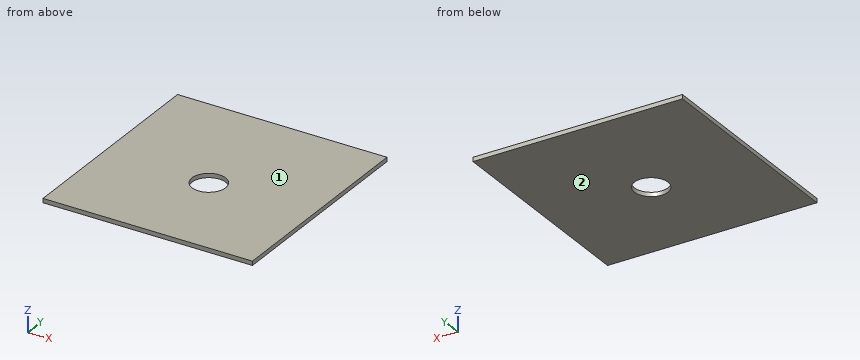
```python
from build123d import *

# Parameters (mm, degrees)
SKETCH1_W           = 249.6
SKETCH1_H           = 257.4
BOSS_EXTRUDE1_DEPTH = 5
SKETCH2_R           = 20
CUT_EXTRUDE1_DEPTH  = 6


with BuildPart() as part:
    # Sketch1 → Boss-Extrude1 (new body)
    with BuildSketch(Plane.XY):
        with Locations((124.8, -128.7)):
            Rectangle(SKETCH1_W, SKETCH1_H)
    extrude(amount=BOSS_EXTRUDE1_DEPTH)

    # Sketch2 → Cut-Extrude1 (cut, through all)
    with BuildSketch(Plane.XY.offset(5)):
        with Locations((125, -140.910978413)):
            Circle(SKETCH2_R)
    extrude(amount=-CUT_EXTRUDE1_DEPTH, mode=Mode.SUBTRACT)


solid = part.part
```
Here's how the part is built. I have some questions about the finished solid (model axes, mm). Face numbers are marked on the shaded views. Give positions to 0.01 mm unless a question says otherwise; leave off trailing zeros. Write each loop counter-clockwise with the first axis right and the second up, starting at its lowest first coordinate (ties: lowest second). Pieces come first, ordered by that corner, then holes. Notation, with made-up numbers: (-35.5, 63) -> (10.5, 63) arc R15 ccw to (10.5, 91) -> close; hole circle Ø8 at (5, 16). An arc over 180 degrees is marked (long way). Use one line per item in the form item = value.
1) Suppose I cut it at C-C (z = 1.2). Please give me the cut outline in (x, y).
Verdict:
outline = (0, -257.4) -> (249.6, -257.4) -> (249.6, 0) -> (0, 0) -> close; hole circle Ø40 at (125, -140.91)
2) We'd pull the mould along Z, two halves only. Please class the marked faces 1 and 2: +Z half, -Z half, draft (parallel to the pull), parting line (faces both ways), or undercut.
Verdict:
face_1 = +Z half
face_2 = -Z half
3) Suppose I cut it at A-A (x = 125). Please give me the cut outline in (y, z).
Verdict:
outline = (-257.4, 0) -> (-160.91, 0) -> (-160.91, 5) -> (-257.4, 5) -> close; (-120.91, 0) -> (0, 0) -> (0, 5) -> (-120.91, 5) -> close
4) If I drill on L1, parallel to Y at x = 125, z = 2.05; L2, parallel to X at y = -129, z = 1.8; L3, parallel to Y at x = 137, z = 1.75, over which ranges is the centre line in solid material (lowest first)? Write a range as [from, to].
Verdict:
L1 = [-257.4, -160.91], [-120.91, 0]
L2 = [0, 108.93], [141.07, 249.6]
L3 = [-257.4, -156.91], [-124.91, 0]
5) Suppose I cut it at B-B (y = -148). Please give me the cut outline in (x, z), and give its area (3 significant figures).
Verdict:
outline = (0, 0) -> (106.3, 0) -> (106.3, 5) -> (0, 5) -> close; (143.7, 0) -> (249.6, 0) -> (249.6, 5) -> (143.7, 5) -> close
area = 1,060 mm2
